Source: CAD feature listing. Evaluate the final solid. Frame: model axes, mm. A direction names the side the tool comes from. Coordinates: 2 decimals unless noted, no trailing zeros. Loops run counter-clockwise (first coordinate to the right, second up) from the corner with the lowest first, then second, coordinate; pieces in that order, holes last. Notation, with made-up numbers: M -8.5,-35 L 4.5,-35 A13 cw 4.5,-27 Z; hole C -12.75,-13 d7. An arc over 180 degrees is marked long. Write each question's results on one line, items separated by ' | '. Start each with the question number.
from build123d import *

# Parameters (mm, degrees)
F0_W      = 76.2
F0_H      = 76.2
F0_R      = 19.05
F1_DEPTH  = 76.2
F2_R      = 12.7
F3_DEPTH  = 76.2
F4_R      = 25.4
F5_DEPTH  = 76.2
F6_R      = 22.225
F6_R_2    = 19.05
F7_DEPTH  = 38.1
F8_R      = 28.575
F9_DEPTH  = 38.1
F10_R     = 15.875
F11_DEPTH = 38.1


with BuildPart() as f1:
    # F0 (on Front) → F1 (new body)
    with BuildSketch(Plane.XZ):
        Rectangle(F0_W, F0_H)
        Circle(F0_R, mode=Mode.SUBTRACT)
    extrude(amount=F1_DEPTH)

    # F2 (on face) → F3 (cut)
    with BuildSketch(Plane.YZ.offset(38.1)):
        with Locations((-38.1, 0)):
            Circle(F2_R)
    extrude(amount=-F3_DEPTH, mode=Mode.SUBTRACT)

    # F4 (on face) → F5 (cut)
    with BuildSketch(Plane(origin=(0, 0, -38.1), x_dir=(1, 0, 0), z_dir=(0, 0, -1))):
        with Locations((0, 38.1)):
            Circle(F4_R)
    extrude(amount=-F5_DEPTH, mode=Mode.SUBTRACT)

    # F6 (on face) → F7 (cut)
    with BuildSketch(Plane(origin=(0, 0, 0), x_dir=(-1, 0, 0), z_dir=(0, 1, 0))):
        Circle(F6_R)
        Circle(F6_R_2, mode=Mode.SUBTRACT)
    extrude(amount=-F7_DEPTH, mode=Mode.SUBTRACT)

    # F8 (on face) → F9 (cut)
    with BuildSketch(Plane(origin=(0, 0, -38.1), x_dir=(1, 0, 0), z_dir=(0, 0, -1))):
        with Locations((0, 38.1)):
            Circle(F8_R)
    extrude(amount=-F9_DEPTH, mode=Mode.SUBTRACT)

    # F10 (on face) → F11 (cut)
    with BuildSketch(Plane.YZ.offset(38.1)):
        with Locations((-38.1, 0)):
            Circle(F10_R)
    extrude(amount=-F11_DEPTH, mode=Mode.SUBTRACT)


solid = f1.part
Item 1: First-contact query: pin 1 Ø1 at (x, z) = (12.5, -13) entering from -Y; pin 2 Ø0.5 at (x, y) = (22.5, -21.5) entering from -Z. Flat tips, straight axial feed; report the tip coordinate or a pass-through.
Item 2: Line query: probe 1 along Z at (x, y) = (-31.5, -38.1); probe 2 along X at (y, z) = (-38.1, 28); probe 3 along Y at (x, z) = (-33, 0). Output: solid intervals per line, ascending.
Item 3: Cut plane C-C (z = 3.5). Output: boundary loops of the cut face in (x, y).
Item 4: Cut plane D-D (y = -56). Output: boundary loops of the cut face in (x, z).
Item 5: Cut plane A-A (y = -38.1). Output: boundary loops of the cut face in (x, z) (3 decimals).
Item 6: Mould query, pull axis Z, two halves, no side actions, for faces 4 (the flat face through (-38.1, -38, -17)), 5 (the flat face through (-24, -23, 0)), 6 (the cylindrical face through (-31.725, -39.753, 12.592)). Classes: +Z half, -Z half, draft (parallel to the pull), parting line (faces both ways), or undercut.
Item 7: Access query for faces 1 (the cylindrical face through (31.12, -40.17, 15.74)), 2 (the cylindrical face through (-21.061, -57.412, -23.55)), 3 (the cylindrical face through (2.893, -9.776, 22.036)). Directions: +Z, -Z, +X, -X, +Y, -Y. A direction counts if a zero-diameter tool reaches every point of the face in a straight line with its end or side. Return the directions, or none.
Item 8: Cut plane B-B (x = 0). Output: boundary loops of the cut face in (y, z) (3 decimals), then the cut area to 3 significant figures.
Response values:
1) pin 1: passes through | pin 2: stops at z = 0
2) probe 1: z = -38.1 to -12.7, 12.7 to 38.1 | probe 2: x = -38.1 to -25.4, 25.4 to 38.1 | probe 3: y = -76.2 to -50.8, -25.4 to 0
3) outline: M -38.1,-76.2 L -18.73,-76.2 L -18.73,-55.26 A25.4 cw -22.27,-50.31 L -38.1,-50.31 Z; M -38.1,-25.89 L -22.27,-25.89 A25.4 cw -21.95,-25.31 L -21.95,0 L -38.1,0 Z; M 18.73,-76.2 L 38.1,-76.2 L 38.1,-53.58 L 20.13,-53.58 A25.4 cw 18.73,-55.26 Z; M 21.95,-22.62 L 38.1,-22.62 L 38.1,0 L 21.95,0 Z
4) outline: M -38.1,-38.1 L -22.27,-38.1 L -22.27,0 L -19.05,0 A19.05 cw -18.02,6.18 L -18.02,38.1 L -38.1,38.1 Z; M 18.02,6.18 A19.05 cw 19.05,0 L 22.27,0 L 22.27,-38.1 L 38.1,-38.1 L 38.1,38.1 L 18.02,38.1 Z
5) outline: M -38.1,-38.1 L -28.575,-38.1 L -28.575,-12.7 L -38.1,-12.7 Z; M -38.1,12.7 L -25.4,12.7 L -25.4,38.1 L -38.1,38.1 Z; M 25.4,15.875 L 38.1,15.875 L 38.1,38.1 L 25.4,38.1 Z; M 28.575,-38.1 L 38.1,-38.1 L 38.1,-15.875 L 28.575,-15.875 Z
6) face 4: draft | face 5: -Z half | face 6: undercut
7) face 1: +X | face 2: -Z | face 3: +Y
8) outline: M -76.2,-38.1 L -66.675,-38.1 L -66.675,-19.05 L -76.2,-19.05 Z; M -76.2,19.05 L -63.5,19.05 L -63.5,38.1 L -76.2,38.1 Z; M -12.7,22.225 L 0,22.225 L 0,38.1 L -12.7,38.1 Z; M -9.525,-38.1 L 0,-38.1 L 0,-22.225 L -9.525,-22.225 Z | area: 776 mm2
